Verification items for the finished model (mm, model axes). A direction names the side the tool comes from. Give positions to 0.01 mm unless a question says otherwise; leave off trailing zeros. Order: outer loops, then holes, each group sorted by start corner. A loop starts at its lowest first (then second) coordinate and runs counter-clockwise, first axis right, second up. Notation, with made-up numbers: (17, 21) - (36, 21) arc R17 ccw to (36, 53) - close; hole circle Ø3 at (4.5, 36.5). An arc over 180 degrees is marked (long way). Answer as a JSON object with one key per item and string values.
```python
from build123d import *

# Parameters (mm, degrees)
SKETCH1_W                 = 228.6
SKETCH1_H                 = 139.7
BOSS_EXTRUDE1_DEPTH       = 6.35
SKETCH5_W                 = 6.35
SKETCH5_H                 = 25.4
CUT_EXTRUDE4_DEPTH        = 6.35
SKETCH6_W                 = 25.4
SKETCH6_H                 = 6.35
CUT_EXTRUDE5_DEPTH        = 6.35
LPATTERN5_COUNT           = 3
LPATTERN5_PITCH           = 50.8
LPATTERN5_COUNT_DIR2      = 2
LPATTERN5_PITCH_DIR2      = 222.25
LPATTERN6_COUNT           = 5
LPATTERN6_PITCH           = 50.8
LPATTERN6_COUNT_DIR2      = 2
LPATTERN6_PITCH_DIR2      = 120.65
SKETCH7_W                 = 6.35
SKETCH7_H                 = 19.05
CUT_EXTRUDE6_DEPTH        = 6.35
SKETCH8_W                 = 6.35
SKETCH8_H                 = 19.05
CUT_EXTRUDE7_DEPTH        = 6.35
F_4_CLEARANCE_HOLE1_D     = 3.2639
F_4_CLEARANCE_HOLE1_DEPTH = 10.16
F_4_CLEARANCE_HOLE1_TIP   = 0.980574487
SKETCH11_R                = 0.55
SKETCH11_R_2              = 9.1
CUT_EXTRUDE8_DEPTH        = 6.35
SKETCH12_R                = 1.75
CUT_EXTRUDE9_DEPTH        = 6.35
SKETCH13_W                = 24.5
SKETCH13_H                = 24.5
CUT_EXTRUDE10_DEPTH       = 6.35


with BuildPart() as part:
    # Sketch1 → Boss-Extrude1 (new body)
    with BuildSketch(Plane.XY):
        with Locations((114.3, 69.85)):
            Rectangle(SKETCH1_W, SKETCH1_H)
    extrude(amount=BOSS_EXTRUDE1_DEPTH)

    # Sketch5 → Cut-Extrude4 (cut)
    with BuildSketch(Plane.XY.offset(6.35)):
        with Locations((3.175, 12.7)):
            Rectangle(SKETCH5_W, SKETCH5_H)
    cut_extrude4 = extrude(amount=-CUT_EXTRUDE4_DEPTH, mode=Mode.SUBTRACT)

    # Sketch6 → Cut-Extrude5 (cut)
    with BuildSketch(Plane.XY.offset(6.35)):
        with Locations((12.7, 3.175)):
            Rectangle(SKETCH6_W, SKETCH6_H)
    cut_extrude5 = extrude(amount=-CUT_EXTRUDE5_DEPTH, mode=Mode.SUBTRACT)

    # LPattern5: Cut-Extrude4 3 × 2
    with Locations(*[(j * LPATTERN5_PITCH_DIR2, i * LPATTERN5_PITCH, 0) for i in range(LPATTERN5_COUNT) for j in range(LPATTERN5_COUNT_DIR2) if (i, j) != (0, 0)]):
        add(cut_extrude4, mode=Mode.SUBTRACT)

    # LPattern6: Cut-Extrude5 5 × 2
    with Locations(*[(i * LPATTERN6_PITCH, j * LPATTERN6_PITCH_DIR2, 0) for i in range(LPATTERN6_COUNT) for j in range(LPATTERN6_COUNT_DIR2) if (i, j) != (0, 0)]):
        add(cut_extrude5, mode=Mode.SUBTRACT)

    # Sketch7 → Cut-Extrude6 (cut)
    with BuildSketch(Plane.XY.offset(6.35)):
        with Locations((3.175, 130.175)):
            Rectangle(SKETCH7_W, SKETCH7_H)
    extrude(amount=-CUT_EXTRUDE6_DEPTH, mode=Mode.SUBTRACT)

    # Sketch8 → Cut-Extrude7 (cut)
    with BuildSketch(Plane.XY.offset(6.35)):
        with Locations((225.425, 130.175)):
            Rectangle(SKETCH8_W, SKETCH8_H)
    extrude(amount=-CUT_EXTRUDE7_DEPTH, mode=Mode.SUBTRACT)

    # #4 Clearance Hole1
    with Locations(Plane.XY.offset(6.35)):
        with Locations((38.1, 123.825), (190.5, 123.825)):
            Hole(F_4_CLEARANCE_HOLE1_D / 2, depth=F_4_CLEARANCE_HOLE1_DEPTH)
            with Locations((0, 0, -(F_4_CLEARANCE_HOLE1_DEPTH + F_4_CLEARANCE_HOLE1_TIP / 2))):  # 118° drill point
                Cone(0, F_4_CLEARANCE_HOLE1_D / 2, F_4_CLEARANCE_HOLE1_TIP, mode=Mode.SUBTRACT)

    # Sketch11 → Cut-Extrude8 (cut)
    with BuildSketch(Plane.XY.offset(6.35)):
        with Locations((177.8, 72.6)):
            Circle(SKETCH11_R)
        with Locations((177.8, 63.5)):
            Circle(SKETCH11_R_2)
    extrude(amount=-CUT_EXTRUDE8_DEPTH, mode=Mode.SUBTRACT)

    # Sketch12 → Cut-Extrude9 (cut)
    with BuildSketch(Plane.XY.offset(6.35)):
        with Locations((107, 88.9)):
            Circle(SKETCH12_R)
        with Locations((147, 88.9)):
            Circle(SKETCH12_R)
        with BuildLine():
            Line((116.75, 100.15), (137.25, 100.15))
            ThreePointArc((137.25, 100.15), (140.785533906, 98.685533906), (142.25, 95.15))
            Line((142.25, 95.15), (142.25, 82.65))
            ThreePointArc((142.25, 82.65), (140.785533906, 79.114466094), (137.25, 77.65))
            Line((137.25, 77.65), (116.75, 77.65))
            ThreePointArc((116.75, 77.65), (113.214466094, 79.114466094), (111.75, 82.65))
            Line((111.75, 82.65), (111.75, 95.15))
            ThreePointArc((111.75, 95.15), (113.214466094, 98.685533906), (116.75, 100.15))
        make_face()
    extrude(amount=-CUT_EXTRUDE9_DEPTH, mode=Mode.SUBTRACT)

    # Sketch13 → Cut-Extrude10 (cut)
    with BuildSketch(Plane.XY.offset(6.35)):
        with Locations((127.45, 44)):
            Rectangle(SKETCH13_W, SKETCH13_H)
    extrude(amount=-CUT_EXTRUDE10_DEPTH, mode=Mode.SUBTRACT)


solid = part.part
```
(1) Section check C-C (x = 171.5). Record the cut outline in (y, z), then the cut area to 3 significant figures.
Computed values:
{"outline": "(6.35, 0) - (56.93, 0) - (56.93, 6.35) - (6.35, 6.35) - close; (70.07, 0) - (120.65, 0) - (120.65, 6.35) - (70.07, 6.35) - close; (127, 0) - (139.7, 0) - (139.7, 6.35) - (127, 6.35) - close", "area": "723 mm²"}
(2) Section check B-B (y = 63.5). Record the cut outline in (x, z), then the cut area to 3 significant figures.
Computed values:
{"outline": "(6.35, 0) - (168.7, 0) - (168.7, 6.35) - (6.35, 6.35) - close; (186.9, 0) - (222.25, 0) - (222.25, 6.35) - (186.9, 6.35) - close", "area": "1,260 mm²"}
(3) Gauge pin test, flat ends, axial feed: pin 1 Ø1.9 at (y, z) = (4.5, 4.5) entering from +X; pin 2 Ø1.9 at (x, z) = (18, 2.5) entering from -Y; pin 3 Ø1.9 at (x, z) = (3.5, 2.5) entering from -Y. Record the tip position at first contact, or that the pin passes through.
Computed values:
{"pin 1": "stops at x = 203.2", "pin 2": "stops at y = 6.35", "pin 3": "stops at y = 25.4"}
(4) Access from +Z, -Z, +X, -X, +Y, -Y to the whole of each face (thin tool, end or side, straight path). Record for faces 5 (the flat face through (3, 76.2, 3)), 6 (the flat face through (222.25, 133, 3)), 7 (the flat face through (225, 76.2, 3)), 8 (the flat face through (50.8, 3, 3)), 9 (the flat face through (142.25, 89, 3)).
Computed values:
{"face 5": "+Z, -Z, -X", "face 6": "+Z, -Z, +X, +Y", "face 7": "+Z, -Z, +X", "face 8": "+Z, -Z, -Y", "face 9": "+Z, -Z"}
(5) Section check D-D (z = 4.5). Count the separate pieces of the cut face and the enclosed holes in it, then the cut area to 3 significant figures.
Computed values:
{"separate pieces": "1", "enclosed holes": "10", "area": "27,800 mm²"}
(6) Release check for a two-part mould opening along X. For faces 1 (the flat face through (113, 71, 6.35)), 2 (the flat face through (165, 127, 3)), 3 (the flat face through (222.25, 63, 3)), 4 (the flat face through (0, 38, 3)) record: pulls with the +X half, pulls with the -X half, needs draft (parallel to the pull), parting line crosses it, or undercut.
Computed values:
{"face 1": "needs draft", "face 2": "undercut", "face 3": "pulls with the +X half", "face 4": "pulls with the -X half"}
(7) Section check A-A (x = 121). Record the cut outline in (y, z).
Computed values:
{"outline": "(6.35, 0) - (31.75, 0) - (31.75, 6.35) - (6.35, 6.35) - close; (56.25, 0) - (77.65, 0) - (77.65, 6.35) - (56.25, 6.35) - close; (100.15, 0) - (120.65, 0) - (120.65, 6.35) - (100.15, 6.35) - close; (127, 0) - (139.7, 0) - (139.7, 6.35) - (127, 6.35) - close"}
(8) Material ranges on line 1 along X through (y, z) = (123.5, 4.5); line 2 along Y through (x, z) = (128.5, 1.25); line 3 along X through (y, z) = (88.9, 2.75), recorded low to high. Write a range as [from, to].
Computed values:
{"line 1": "x = [25.4, 36.5], [39.7, 50.8], [76.2, 101.6], [127, 152.4], [177.8, 188.9], [192.1, 203.2]", "line 2": "y = [0, 31.75], [56.25, 77.65], [100.15, 139.7]", "line 3": "x = [0, 105.25], [108.75, 111.75], [142.25, 145.25], [148.75, 228.6]"}
